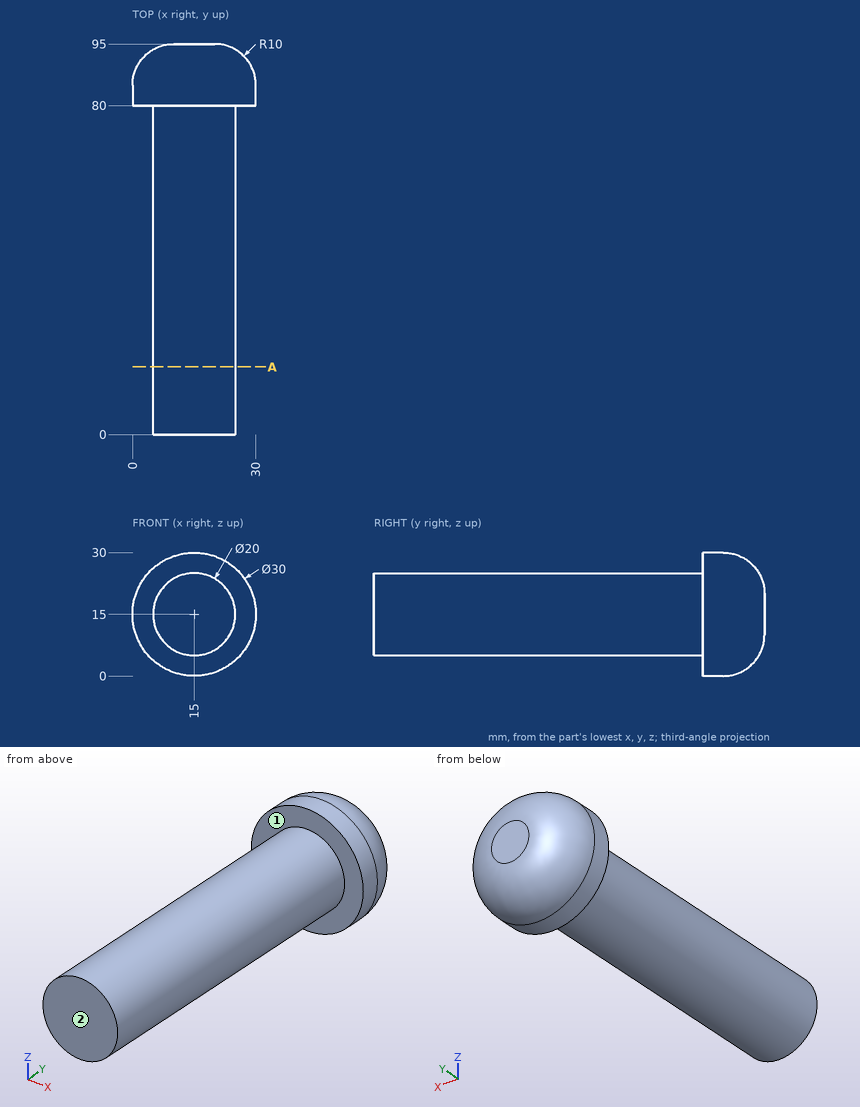
Could you check a few things on this drawing? It's one solid part, dimensions in mm from its lowest x, y, z. A direction names the side the tool comes from. Coordinates: 2 decimals unless noted, no trailing zeros. Order: outer loops, then holes, each group sorted by start corner. A loop starts at its lowest first (then second) coordinate and runs counter-clockwise, first axis right, second up.
1) Will these pins go through, and if not, where does the flat tip stop? pin 1 (1.5 mm diameter, centred on y = 39, z = 8.5, fed in from -X); pin 2 (5 mm diameter, centred on x = 5, z = 21, fed in from -Y); pin 3 (12 mm diameter, centred on y = 58, z = 25, fed in from -X); pin 4 (12 mm diameter, centred on y = 49.5, z = 14.5, fed in from -X).
2) I need wall thicknesses on line 1 (X direction, y = 85.5, z = 22.75); line 2 (Y direction, x = 13, z = 26.5); line 3 (Z direction, x = 4.75, y = 86). Which ranges of each line are inside material? Lowest first, please.
3) Imagine slicing it at A-A on y = 16.5. List the corners of the cut face in (x, z) for me.
4) Which directions (+Z, -Z, +X, -X, +Y, -Y) give clear straight access to the entire face, cutting with the end or side of a thin tool? Please do the marked faces 1 and 2.
Response values:
1. pin 1: stops at x = 6.82
1. pin 2: stops at y = 0
1. pin 3: stops at x = 5.83
1. pin 4: stops at x = 5
2. line 1: x = 2.17 to 27.83
2. line 2: y = 80 to 92.45
2. line 3: z = 4.12 to 25.88
3. outline: circle Ø20 at (15, 15)
4. face 1: -Y
4. face 2: +Z, -Z, +X, -X, -Y
